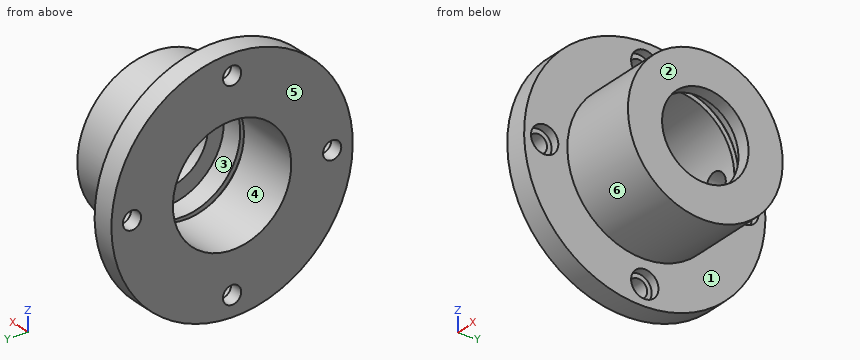
from build123d import *

# Parameters (mm, degrees)
SKETCH1_R           = 26.5
SKETCH1_R_2         = 2
BOSS_EXTRUDE1_DEPTH = 11.5
SKETCH2_R           = 26.5
SKETCH2_R_2         = 17
SKETCH2_R_3         = 2
CUT_EXTRUDE1_DEPTH  = 18
SKETCH3_R           = 13
CUT_EXTRUDE2_DEPTH  = 20
SKETCH4_R           = 9.5
CUT_EXTRUDE3_DEPTH  = 20
SKETCH5_R           = 14
CUT_EXTRUDE4_DEPTH  = 0.55
SKETCH6_R           = 3
CUT_EXTRUDE5_DEPTH  = 33
SKETCH9_R           = 3
CUT_EXTRUDE7_DEPTH  = 2


with BuildPart() as part:
    # Sketch1 → Boss-Extrude1 (new body, symmetric)
    with BuildSketch(Plane(origin=(0, 0, 0), x_dir=(0, 0, -1), z_dir=(1, 0, 0))):
        Circle(SKETCH1_R)
        with Locations((0, -21.987670406)):
            Circle(SKETCH1_R_2, mode=Mode.SUBTRACT)
        with Locations((-21.987670406, 0)):
            Circle(SKETCH1_R_2, mode=Mode.SUBTRACT)
        with Locations((0, 21.987670406)):
            Circle(SKETCH1_R_2, mode=Mode.SUBTRACT)
        with Locations((21.987670406, 0)):
            Circle(SKETCH1_R_2, mode=Mode.SUBTRACT)
    extrude(amount=BOSS_EXTRUDE1_DEPTH, both=True)

    # Sketch2 → Cut-Extrude1 (cut)
    with BuildSketch(Plane(origin=(11.5, 0, 0), x_dir=(0, 0, -1), z_dir=(1, 0, 0))):
        Circle(SKETCH2_R)
        Circle(SKETCH2_R_2, mode=Mode.SUBTRACT)
        with Locations((0, -21.987670406)):
            Circle(SKETCH2_R_3, mode=Mode.SUBTRACT)
        with Locations((-21.987670406, 0)):
            Circle(SKETCH2_R_3, mode=Mode.SUBTRACT)
        with Locations((21.987670406, 0)):
            Circle(SKETCH2_R_3, mode=Mode.SUBTRACT)
        with Locations((0, 21.987670406)):
            Circle(SKETCH2_R_3, mode=Mode.SUBTRACT)
    extrude(amount=-CUT_EXTRUDE1_DEPTH, mode=Mode.SUBTRACT)

    # Sketch3 → Cut-Extrude2 (cut)
    with BuildSketch(Plane.ZY.offset(11.5)):
        Circle(SKETCH3_R)
    extrude(amount=-CUT_EXTRUDE2_DEPTH, mode=Mode.SUBTRACT)

    # Sketch4 → Cut-Extrude3 (cut)
    with BuildSketch(Plane.ZY.offset(-8.5)):
        Circle(SKETCH4_R)
    extrude(amount=-CUT_EXTRUDE3_DEPTH, mode=Mode.SUBTRACT)

    # Sketch5 → Cut-Extrude4 (cut, symmetric)
    with BuildSketch(Plane.ZY.offset(-3.1)):
        Circle(SKETCH5_R)
    extrude(amount=CUT_EXTRUDE4_DEPTH, both=True, mode=Mode.SUBTRACT)

    # Sketch6 → Cut-Extrude5 (cut)
    with BuildSketch(Plane(origin=(0, 0, 0), x_dir=(1, 0, 0), z_dir=(0, 1, 0))):
        with Locations((-3, 0)):
            Circle(SKETCH6_R)
    extrude(amount=CUT_EXTRUDE5_DEPTH, mode=Mode.SUBTRACT)

    # Sketch9 → Cut-Extrude7 (cut)
    with BuildSketch(Plane(origin=(-6.5, 0, 0), x_dir=(0, 0, -1), z_dir=(1, 0, 0))):
        with Locations((0, 21.987670406)):
            Circle(SKETCH9_R)
        with Locations((21.987670406, 0)):
            Circle(SKETCH9_R)
        with Locations((0, -21.987670406)):
            Circle(SKETCH9_R)
        with Locations((-21.987670406, 0)):
            Circle(SKETCH9_R)
    extrude(amount=-CUT_EXTRUDE7_DEPTH, mode=Mode.SUBTRACT)


solid = part.part
The listing builds one solid part. Answer for the finished solid, in the listing's coordinates (mm). Face numbers are marked on the shaded views. A direction names the side the tool comes from. Round coordinates to 2 decimals unless told otherwise and drop trailing zeros. Order: outer loops, then holes, each group sorted by start corner. A loop starts at its lowest first (then second) coordinate and runs counter-clockwise, first axis right, second up. Notation, with made-up numbers: (-10, -20.5) -> (23, -20.5) arc R20 cw to (23, 14.5) -> close; hole circle Ø6 at (28.5, 10.25). An arc over 180 degrees is marked (long way). One line per item, written item: value.
Item 1: Given P1, Ø3, axis at y = 0, z = 21.99, coming from the -X side; P2, Ø1, axis at x = -9, y = -3.5, coming from the -Z side; P3, Ø6, axis at x = 5.5, y = 3, coming from the -Z side; P4, Ø3, axis at y = -21, z = -1.5, coming from the +X side, each flat-ended and moving along its own axis, determine where each tip first touches the part or whether it passes through.
Taken from the geometry:
P1: passes through
P2: stops at z = -26.33
P3: stops at z = -17
P4: stops at x = -6.5
Item 2: Find section B-B, the plane y = -4.5. Give the vertices of the cut face in (x, z), then the cut area to 3 significant figures.
Taken from the geometry:
outline: (-11.5, -26.12) -> (-6.5, -26.12) -> (-6.5, -16.39) -> (11.5, -16.39) -> (11.5, -8.37) -> (8.5, -8.37) -> (8.5, -12.2) -> (3.65, -12.2) -> (3.65, -13.26) -> (2.55, -13.26) -> (2.55, -12.2) -> (-11.5, -12.2) -> close; (-11.5, 12.2) -> (2.55, 12.2) -> (2.55, 13.26) -> (3.65, 13.26) -> (3.65, 12.2) -> (8.5, 12.2) -> (8.5, 8.37) -> (11.5, 8.37) -> (11.5, 16.39) -> (-6.5, 16.39) -> (-6.5, 26.12) -> (-11.5, 26.12) -> close
area: 311 mm2
Item 3: Find section A-A, the plane z = -21. Give the vertices of the cut face in (x, y), then the cut area to 3 significant figures.
Taken from the geometry:
outline: (-11.5, -16.16) -> (-6.5, -16.16) -> (-6.5, -2.83) -> (-8.5, -2.83) -> (-8.5, -1.74) -> (-11.5, -1.74) -> close; (-11.5, 1.74) -> (-8.5, 1.74) -> (-8.5, 2.83) -> (-6.5, 2.83) -> (-6.5, 16.16) -> (-11.5, 16.16) -> close
area: 140 mm2
Item 4: Straight lines are drawn through the part: L1, parallel to Y at x = -9.15, z = 0; L2, parallel to X at y = -10, z = 8.5; L3, parallel to X at y = 18, z = 6. For each, find the intervals that lie inside material, in ascending order.
Taken from the geometry:
L1: y = -26.5 to -23.99, -19.99 to -13, 13 to 19.99, 23.99 to 26.5
L2: x = -11.5 to 2.55, 3.65 to 11.5
L3: x = -11.5 to -6.5
Item 5: Find section C-C, the plane x = 1.25. Give the vertices of the cut face in (y, z).
Taken from the geometry:
outline: circle Ø34 at (0, 0); hole circle Ø26 at (0, 0)
Item 6: Find section D-D, the plane z = 0. State how many separate pieces and enclosed holes the cut face has, then the cut area to 3 significant figures.
Taken from the geometry:
separate pieces: 5
enclosed holes: 0
area: 226 mm2
Item 7: For the marked faces 1 and 2, determine the directions among +Z, -Z, +X, -X, +Y, -Y from which every point of the face is accessible in a straight line to the end or side of a thin tool.
Taken from the geometry:
face 1: +X
face 2: +Z, -Z, +X, +Y, -Y
Item 8: For a pull along Y with two mould halves and no side action, classify the marked faces 3, 4, 5 and 6 as released by +Y, released by -Y, zero draft, split by the parting line, or undercut.
Taken from the geometry:
face 3: undercut
face 4: undercut
face 5: zero draft
face 6: split by the parting line
